Autodesk Inventor part; units mm, degrees
ref_plane "YZ Plane" through (0, 0, 0) normal (1, 0, 0) x (0, 1, 0)
ref_plane "XZ Plane" through (0, 0, 0) normal (0, 1, 0) x (-1, 0, 0)
ref_plane "XY Plane" through (0, 0, 0) normal (0, 0, 1) x (1, 0, 0)
sketch "Sketch1" plane through (0, 0, 0) normal (0, 0, 1) x (1, 0, 0)
  line L0 (8.25, 5) -> (-8.25, 5)
  line L1 (-8.25, 5) -> (-8.25, -5)
  line L2 (-8.25, -5) -> (8.25, -5)
  line L3 (8.25, -5) -> (8.25, 5)
  point P0 (0, 0)
  dimension "d19" = 10
  dimension "d36" = 16.5
  dimension "d37" = 5
extrude "Box" add sketch "Sketch1" along normal blind 6.927 and the other way blind 6.223
sketch "Sketch3" plane through (0, 0, -6.223) normal (0, 0, -1) x (-1, 0, 0)
  line L0 (-5.08, 0) -> (5.08, 0) construction
  line L1 (-4.75, 0) -> (4.75, 0) construction
  circle A0 centre (0, 0) radius 2
  dimension "d35" = 4
extrude "Slot" cut sketch "Sketch3" against normal blind 6.605
sketch "Sketch4" plane through (0, 0, -6.223) normal (0, 0, -1) x (-1, 0, 0)
  circle A0 centre (-2.96, 3.0769) radius 1.45
  line L0 (8.25, 5) -> (-8.25, 5)
  circle A1 centre (0, 0) radius 2
  line L1 (-8.25, 5) -> (-8.25, -5)
  dimension "d32" = 2.9
  dimension "d34" = 1.9231
  dimension "d39" = 5.29
  dimension "d40" = 5
extrude "MountingHole" cut sketch "Sketch4" against normal blind 15 contours A0
pattern_linear "Mounting Holes" count 2 spacing 5.92 along (-1, 0, 0) count 2 spacing 6.154 along (0, -1, 0) of "MountingHole"
sketch "Sketch6" plane through (-8.25, 5, 6.927) normal (0, 1, 0) x (1, 0, 0)
  circle A0 centre (8.25, 9.65) radius 1.105
  line L0 (0, 13.15) -> (16.5, 13.15)
  dimension "d20" = 2.21
  dimension "d46" = 3.5
extrude "CentralSMAHole" cut sketch "Sketch6" against normal blind 12
sketch "Sketch8" plane through (-8.25, 5, 6.927) normal (0, 1, 0) x (1, 0, 0)
  circle A0 centre (14.36, 9.65) radius 1.295
  line L0 (0, 13.15) -> (16.5, 13.15)
  dimension "d23" = 2.59
  dimension "d45" = 3.5
extrude "SMAMounting" cut sketch "Sketch8" against normal blind 12
pattern_linear "SMAMountingHoles" count 2 spacing 12.22 along (-1, 0, 0) of "SMAMounting"
equation "\"d34\" = 0.384615 * d40"
properties part number "NewSinkV4"
Model file for the job. Use its own axes, mm. A direction names the side the tool comes from. Round coordinates to 2 decimals unless told otherwise and drop trailing zeros. Write each loop counter-clockwise with the first axis right and the second up, starting at its lowest first coordinate (ties: lowest second). Pieces come first, ordered by that corner, then holes. Notation, with made-up numbers: (-11, 50) - (9, 50) arc R30 cw to (9, 89) - close; hole circle Ø6 at (30.5, -38). An arc over 180 degrees is marked (long way). One line per item, written item: value.
(1) Cut at B-B, the plane z = 0.75. Give the cut face in (x, y).
Values follow:
outline: (-8.25, -5) - (8.25, -5) - (8.25, 5) - (-8.25, 5) - close; hole circle Ø2.9 at (-2.96, -3.08); hole circle Ø2.9 at (-2.96, 3.08); hole circle Ø2.9 at (2.96, -3.08); hole circle Ø2.9 at (2.96, 3.08)
(2) Wall check: probe 1 along Y at (x, z) = (3, -5.25); probe 2 along Z at (x, y) = (0, 3.3); probe 3 along X at (y, z) = (3.75, -4.75). Give the ranges that are in metal, low to high.
Values follow:
probe 1: y = -5 to -4.53, -1.63 to 1.63, 4.53 to 5
probe 2: z = -6.22 to -3.83, -1.62 to 6.93
probe 3: x = -8.25 to -4.24, -1.68 to 1.68, 4.24 to 8.25
(3) Cut at C-C, the plane y = 2.5. Give the cut face in (x, z) (3 decimals).
Values follow:
outline: (-8.25, -6.223) - (-4.29, -6.223) - (-4.29, 6.927) - (-8.25, 6.927) - close; (-1.63, -6.223) - (1.63, -6.223) - (1.63, 6.927) - (-1.63, 6.927) - close; (4.29, -6.223) - (8.25, -6.223) - (8.25, 6.927) - (4.29, 6.927) - close; hole circle Ø2.59 at (-6.11, -2.723); hole circle Ø2.21 at (0, -2.723); hole circle Ø2.59 at (6.11, -2.723)
(4) Two-plate mould, pull along Z, no slides. Class faces 1 (the cylindrical face through (-7.14, 0.07, -1.94)), 2 (the flat face through (0, 0, 0.382)), 3 (the cylindrical face through (1.577, 3.512, 0.26)), 4 (the cylindrical face through (5.08, 0.07, -1.94)): pulls with the +Z half, pulls with the -Z half, needs draft (parallel to the pull), parting line crosses it, or undercut.
Values follow:
face 1: undercut
face 2: pulls with the -Z half
face 3: needs draft
face 4: undercut
(5) Drop flat-ended pins along their axis: P1, Ø4.5, axis at x = 0.5, y = 0, coming from the -Z side; P2, Ø1.3, axis at x = 0, z = -2.723, coming from the -Y side; P3, Ø3, axis at x = 0, y = 0, coming from the -Z side. Give the stop position or say it passes through.
Values follow:
P1: stops at z = -6.22
P2: passes through
P3: stops at z = 0.38
(6) Cut at A-A, the plane x = 2.96. Give the cut face in (y, z), plus the area to 3 significant figures.
Values follow:
outline: (-5, -6.22) - (-4.53, -6.22) - (-4.53, 6.93) - (-5, 6.93) - close; (-1.63, -6.22) - (1.63, -6.22) - (1.63, 6.93) - (-1.63, 6.93) - close; (4.53, -6.22) - (5, -6.22) - (5, 6.93) - (4.53, 6.93) - close
area: 55.2 mm²
(7) 3-axis set-ups, long thin cutter, end or side, ignore diameter. For faces 5 (the cylindrical face through (1.474, 1.352, -2.967)), 6 (the flat face through (-8.25, 0, 0)): which of +Z, -Z, +X, -X, +Y, -Y reach the whole face in a straight line?
Values follow:
face 5: -Z
face 6: +Z, -Z, -X, +Y, -Y
(8) Cut at D-D, the plane x = 6.11. Give the cut face in (y, z).
Values follow:
outline: (-5, -6.22) - (5, -6.22) - (5, -4.02) - (-5, -4.02) - close; (-5, -1.43) - (5, -1.43) - (5, 6.93) - (-5, 6.93) - close
